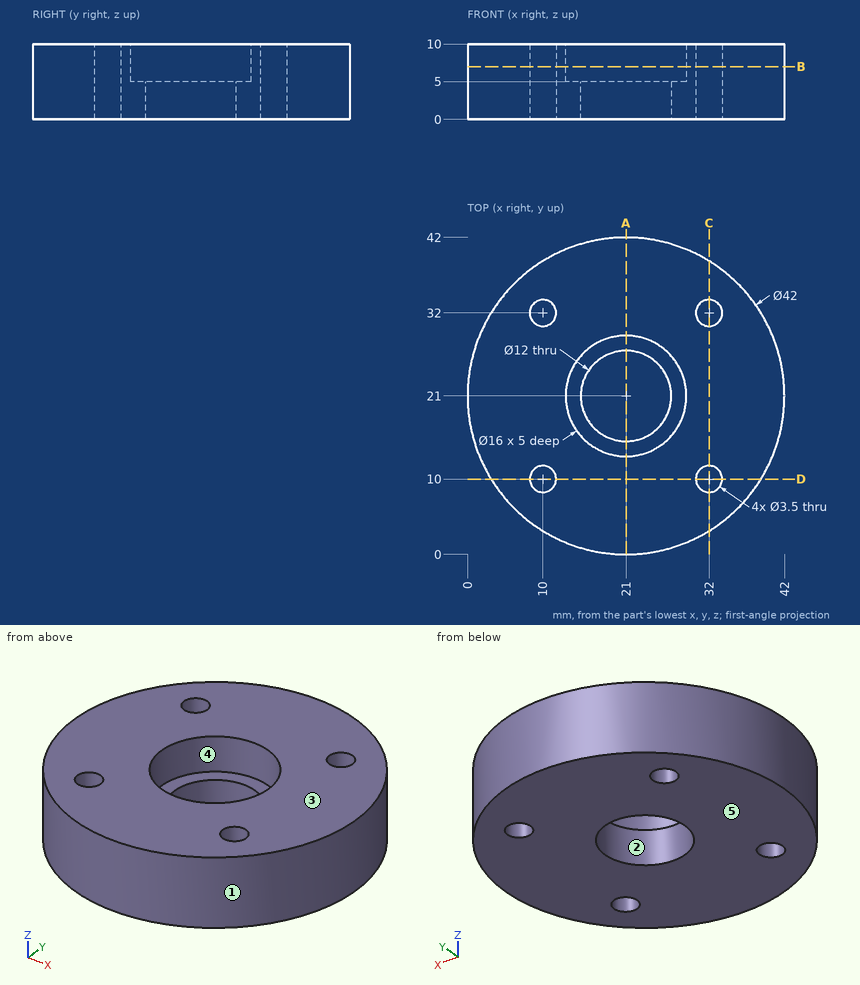
Here's the drawing with two shaded views (mm, measured from the low corner). I have some questions. A direction names the side the tool comes from. Coordinates: 2 decimals unless noted, no trailing zeros. Write each loop counter-clockwise with the first axis right and the second up, starting at its lowest first coordinate (ties: lowest second). Pieces come first, ordered by that corner, then holes. Notation, with made-up numbers: M 85,60.25 L 129,60.25 A23 ccw 129,86.25 Z; hole C -28.75,1.5 d4. An arc over 180 degrees is marked long. Write item = value, one per line. Start each with the question number.
Q1. If we section it at C-C, the plane x = 32: Write out the boundary of the cut face in (y, z), then the cut area to 3 significant figures.
Q2. If I drill on L1, parallel to Y at x = 10, z = 5.5; L2, parallel to X at y = 10.5, z = 2.5; L3, parallel to Y at x = 23, z = 7.75, over which ranges is the centre line in solid material (lowest first)? Write a range as [from, to].
Q3. On a 3-axis mill with a long thin cutter (end or side, diameter ignored), from which of +Z, -Z, +X, -X, +Y, -Y can I reach the whole of each face in a straight line? I mean the marked faces 4 and 5. Say none if no direction works.
Q4. I'm going to push flat-ended pins straight in: pin 1 (19 mm diameter, centred on x = 21, y = 21, fed in from +Z); pin 2 (4 mm diameter, centred on y = 5, z = 3.5, fed in from -X); pin 3 (3 mm diameter, centred on x = 10, y = 32, fed in from -Z); pin 4 (3 mm diameter, centred on x = 18.5, z = 4.5, fed in from -Y). Where does each tip first touch, or does it pass through?
Q5. If we section it at A-A, the plane x = 21: Write out the boundary of the cut face in (y, z).
Q6. If we section it at B-B, the plane z = 7: Write out the boundary of the cut face in (x, y).
Q7. Thinking about a two-plate mould opening in Y: for the marked faces 1, 2 and 3, which applies, released by +Y, released by -Y, zero draft, split by the parting line, or undercut?
Check sheet entries:
q1.outline = M 3.11,0 L 8.25,0 L 8.25,10 L 3.11,10 Z; M 11.75,0 L 30.25,0 L 30.25,10 L 11.75,10 Z; M 33.75,0 L 38.89,0 L 38.89,10 L 33.75,10 Z
q1.area = 288 mm²
q2.L1 = [3.11, 8.25], [11.75, 30.25], [33.75, 38.89]
q2.L2 = [2.81, 8.32], [11.68, 30.32], [33.68, 39.19]
q2.L3 = [0.1, 13.25], [28.75, 41.9]
q3.face_4 = +Z
q3.face_5 = -Z, +X, -X, +Y, -Y
q4.pin_1 = 10
q4.pin_2 = 5.35
q4.pin_3 = through
q4.pin_4 = 0.02
q5.outline = M 0,0 L 15,0 L 15,5 L 13,5 L 13,10 L 0,10 Z; M 27,0 L 42,0 L 42,10 L 29,10 L 29,5 L 27,5 Z
q6.outline = C 21,21 d42; hole C 10,10 d3.5; hole C 10,32 d3.5; hole C 21,21 d16; hole C 32,10 d3.5; hole C 32,32 d3.5
q7.face_1 = split by the parting line
q7.face_2 = undercut
q7.face_3 = zero draft
